Here's how the part is built. I have some questions about the finished solid (model axes, mm). A direction names the side the tool comes from. Round coordinates to 2 decimals unless told otherwise and drop trailing zeros. Loops run counter-clockwise (first coordinate to the right, second up) from the corner with the lowest first, then second, coordinate; pieces in that order, holes last. Notation, with made-up numbers: (56, 7.25) - (114, 7.25) arc R20 ccw to (114, 43.25) - close; hole circle Ø9 at (38.25, -0.5). An arc over 180 degrees is marked (long way). Answer as a JSON object with one key per item and string values. Group by question number.
1) If I drill on line 1 along X through (y, z) = (-35.5, 84); line 2 along Z through (x, y) = (14.25, -30.75); line 3 along Z through (x, y) = (4.7, -32), over which ranges is the centre line in solid material (lowest first)? Write a range as [from, to].
2) Which directions (+Z, -Z, +X, -X, +Y, -Y) give clear straight access to the entire face, cutting with the end or side of a thin tool? Please do faces 1 (the face through (23, -33, 101)), 2 (the face through (8, -32, 120)), 3 (the face through (8, -32, 106)).
3) I want a section at A-A, the plane y = -32. Please give me the cut outline in (x, z), then the cut area to 3 significant figures.
4) Will these pins go through, and if not, where does the flat tip stop? P1, Ø4.5, axis at x = 14, z = 118.5, coming from the +Y side; P2, Ø2, axis at x = 18, z = 84, coming from the -Y side; P3, Ø3, axis at y = -30.5, z = 126.5, coming from the +X side.
5) I want a section at D-D, the plane x = 14.75. Please give me the cut outline in (y, z), then the cut area to 3 significant figures.
6) I want a section at B-B, the plane x = 18. Please give me the cut outline in (y, z), then the cut area to 3 significant figures.
7) I want a section at C-C, the plane z = 84. Please give me the cut outline in (x, y), then the cut area to 3 significant figures.
8) If we mould it in two halves opening along Y, with no side actions, what happens to faces 4 (the face through (7, -32, 128.708)), 5 (the face through (16, -38.5, 120)), 6 (the face through (13, -41, 106))? For each: pulls with the +Y half, pulls with the -Y half, needs draft (parallel to the pull), parting line crosses it, or undercut.
from build123d import *

# Parameters (mm, degrees)
CYLINDER075_R          = 1.75
CYLINDER075_DEPTH      = 32
PRISM001_DEPTH         = 10
SKETCH015_R            = 1
SKETCH015_W            = 24
SKETCH015_H            = 13
PAD010_DEPTH           = 30
CYLINDER073_R          = 1.75
CYLINDER073_DEPTH      = 32
CYLINDER073_ROLL_ANGLE = -90
CYLINDER074_R          = 1.75
CYLINDER074_DEPTH      = 32
CYLINDER074_ROLL_ANGLE = -90
BOX054_W               = 19
BOX054_H               = 15
BOX054_DEPTH           = 56
CHAMFER108_SIZE        = 3


with BuildPart() as cilindro016:
    # Cylinder075 → Cylinder075 (new body)
    with BuildSketch(Plane(origin=(-5, 104, 125.85), x_dir=(0, -1, 0), z_dir=(1, 0, 0))):
        Circle(CYLINDER075_R)
    extrude(amount=CYLINDER075_DEPTH)


with BuildPart() as fusion057:
    # Prism001 → Prism001 (new body)
    with BuildSketch(Plane(origin=(6, 104, 125.85), x_dir=(0, -1, 0), z_dir=(1, 0, 0))):
        Polygon((3.3, 0), (1.65, 2.857884), (-1.65, 2.857884), (-3.3, 0), (-1.65, -2.857884), (1.65, -2.857884), align=None)
    extrude(amount=PRISM001_DEPTH)

    # Fusion057: union Cilindro016
    add(cilindro016.part)


with BuildPart() as pad010:
    # Sketch015 → Pad010 (new body)
    with BuildSketch(Plane(origin=(38, -16, 143.25), x_dir=(0, 0, -1), z_dir=(1, 0, 0))):
        with Locations((37, 120)):
            Circle(SKETCH015_R)
        with Locations((9.5, 120)):
            Circle(SKETCH015_R)
        with Locations((23.25, 120)):
            Rectangle(SKETCH015_W, SKETCH015_H)
    extrude(amount=-PAD010_DEPTH)


with BuildPart() as cilindro014:
    # Cylinder073 → Cylinder073 (new body)
    with BuildSketch(Plane.XY):
        Circle(CYLINDER073_R)
    extrude(amount=CYLINDER073_DEPTH)


with BuildPart() as cilindro014_1:
    # Cylinder073 roll: moved
    add(cilindro014.part.rotate(Axis((0, 0, 0), (1, 0, 0)), CYLINDER073_ROLL_ANGLE))


with BuildPart() as cilindro014_2:
    # Cylinder073 placement: moved
    add(cilindro014_1.part.moved(Location((8, 90, 84))))


with BuildPart() as fusion056:
    # Cylinder074 → Cylinder074 (new body)
    with BuildSketch(Plane.XY):
        Circle(CYLINDER074_R)
    extrude(amount=CYLINDER074_DEPTH)


with BuildPart() as fusion056_1:
    # Cylinder074 roll: moved
    add(fusion056.part.rotate(Axis((0, 0, 0), (1, 0, 0)), CYLINDER074_ROLL_ANGLE))


with BuildPart() as fusion056_2:
    # Cylinder074 placement: moved
    add(fusion056_1.part.moved(Location((18, 90, 84))))

    # Fusion056: union Cilindro014
    add(cilindro014_2.part)


with BuildPart() as clone_of_cut100:
    # Box054 → Box054 (new body)
    with BuildSketch(Plane(origin=(4, 98, 80), x_dir=(1, 0, 0), z_dir=(0, 0, 1))):
        with Locations((9.5, 7.5)):
            Rectangle(BOX054_W, BOX054_H)
    extrude(amount=BOX054_DEPTH)

    # Cut098: cut Fusion056
    add(fusion056_2.part, mode=Mode.SUBTRACT)

    # Cut099: cut Pad010
    add(pad010.part, mode=Mode.SUBTRACT)

    # Chamfer108
    chamfer108_edges = [clone_of_cut100.edges().sort_by_distance(p)[0] for p in [
        (13.5, 113, 136),
    ]]
    chamfer(chamfer108_edges, length=CHAMFER108_SIZE)

    # Cut100: cut Fusion057
    add(fusion057.part, mode=Mode.SUBTRACT)


with BuildPart() as part_mirroring007009:
    # Part__Mirroring007009: instance of Clone of Cut100
    add(clone_of_cut100.part.mirror(Plane(origin=(0, 0, 0), x_dir=(1, 0, 0), z_dir=(0, 1, 0))))


with BuildPart() as part_mirroring007009_1:
    # Part__Mirroring007009 placement: moved
    add(part_mirroring007009.part.moved(Location((0, 72, 0))))


solid = part_mirroring007009_1.part
Outcome:
{
 "1": {"line 1": "[4, 6.25], [9.75, 16.25], [19.75, 23]", "line 2": "[80, 108], [132, 136]", "line 3": "[80, 124.1], [127.6, 136]"},
 "2": {"face 1": "+Z, -Z, +X, +Y, -Y", "face 2": "+X, +Y", "face 3": "+X"},
 "3": {"outline": "(4, 80) - (23, 80) - (23, 105.25) - (8, 105.25) - (8, 107.25) - (23, 107.25) - (23, 108) - (8, 108) - (8, 122.99) - (6, 122.99) - (6, 124.1) - (4, 124.1) - close; (4, 127.6) - (6, 127.6) - (6, 128.71) - (8, 128.71) - (8, 132) - (23, 132) - (23, 132.75) - (8, 132.75) - (8, 134.75) - (23, 134.75) - (23, 136) - (4, 136) - close; hole circle Ø3.5 at (8, 84); hole circle Ø3.5 at (18, 84)", "area": "606 mm^2"},
 "4": {"P1": "y = -38.5", "P2": "through", "P3": "x = 8"},
 "5": {"outline": "(-41, 80) - (-26, 80) - (-26, 108) - (-38.5, 108) - (-38.5, 132) - (-26, 132) - (-26, 136) - (-38, 136) - (-41, 133) - close; hole circle Ø2 at (-32, 106.25); hole circle Ø2 at (-32, 133.75)", "area": "529 mm^2"},
 "6": {"outline": "(-41, 80) - (-26, 80) - (-26, 82.25) - (-41, 82.25) - close; (-41, 85.75) - (-26, 85.75) - (-26, 108) - (-38.5, 108) - (-38.5, 132) - (-26, 132) - (-26, 136) - (-38, 136) - (-41, 133) - close; hole circle Ø2 at (-32, 106.25); hole circle Ø2 at (-32, 133.75)", "area": "477 mm^2"},
 "7": {"outline": "(4, -41) - (6.25, -41) - (6.25, -26) - (4, -26) - close; (9.75, -41) - (16.25, -41) - (16.25, -26) - (9.75, -26) - close; (19.75, -41) - (23, -41) - (23, -26) - (19.75, -26) - close", "area": "180 mm^2"},
 "8": {"face 4": "undercut", "face 5": "pulls with the +Y half", "face 6": "pulls with the -Y half"}
}
